Read the model definition and answer for the solid it produces. Units are mm, in the model's axes. A direction names the side the tool comes from. Round coordinates to 2 decimals unless told otherwise and drop trailing zeros. Order: outer loops, then holes, each group sorted by start corner. A loop starts at its lowest first (then second) coordinate and runs counter-clockwise, first axis right, second up.
from build123d import *

# Parameters (mm, degrees)
F0_W     = 18
F0_H     = 43.2
F1_DEPTH = 1.6
F3_DEPTH = 1
F2_W     = 10.35191
F2_H     = 3.05466
F4_DEPTH = 3


with BuildPart() as f1:
    # F0 (on Top) → F1 (new body)
    with BuildSketch(Plane.XY):
        with Locations((0, -1.040964)):
            Rectangle(F0_W, F0_H)
    extrude(amount=F1_DEPTH)

    # F2 (on face) → F3 (join)
    with BuildSketch(Plane.XY.offset(1.6)):
        Polygon((-3.383941, -9.864242), (0, -13.744771), (3.521491, -9.864242), (0, -5.74118), align=None)
    extrude(amount=F3_DEPTH)

    # F2 (on face) → F4 (join)
    with BuildSketch(Plane.XY.offset(1.6)):
        with Locations((0.296766, 17.023522)):
            Rectangle(F2_W, F2_H)
    extrude(amount=F4_DEPTH)


solid = f1.part
Q1. A cutting plane is placed at D-D, the plane x = 1.5. Give the vertices of the cut face in (y, z), plus the area to 3 significant figures.
Outcome:
outline: (-22.64, 0) - (20.56, 0) - (20.56, 1.6) - (18.55, 1.6) - (18.55, 4.6) - (15.5, 4.6) - (15.5, 1.6) - (-7.5, 1.6) - (-7.5, 2.6) - (-12.09, 2.6) - (-12.09, 1.6) - (-22.64, 1.6) - close
area: 82.9 mm2
Q2. A cutting plane is placed at A-A, the plane x = 4.75. Give the vertices of the cut face in (y, z), plus the area to 3 significant figures.
Outcome:
outline: (-22.64, 0) - (20.56, 0) - (20.56, 1.6) - (18.55, 1.6) - (18.55, 4.6) - (15.5, 4.6) - (15.5, 1.6) - (-22.64, 1.6) - close
area: 78.3 mm2
Q3. For faces 4 (the face through (0, 15.496, 3)), 5 (the face through (0, -10, 2.6)), 6 (the face through (5.473, 17, 3)), 7 (the face through (1.74, -11.83, 2.09)), 8 (the face through (1.785, -7.832, 2.093)), determine the directions among +Z, -Z, +X, -X, +Y, -Y from which every point of the face is accessible in a straight line to the end or side of a thin tool.
Outcome:
face 4: +Z, +X, -X
face 5: +Z, +X, -X, -Y
face 6: +Z, +X, +Y, -Y
face 7: +Z, +X, -Y
face 8: +Z, +X
Q4. For a pull along Y with two mould halves and no side action, classify faces 1 (the face through (0, -1, 1.6)), 2 (the face through (-4.879, 17, 3)), 3 (the face through (0, 18.551, 3)) as released by +Y, released by -Y, zero draft, split by the parting line, or undercut.
Outcome:
face 1: undercut
face 2: zero draft
face 3: released by +Y
Q5. A cutting plane is placed at C-C, the plane z = 3.25. Give the vertices of the cut face in (x, y), plus the area to 3 significant figures.
Outcome:
outline: (-4.88, 15.5) - (5.47, 15.5) - (5.47, 18.55) - (-4.88, 18.55) - close
area: 31.6 mm2
Q6. A cutting plane is placed at B-B, the plane y = -9. Give the vertices of the cut face in (x, z).
Outcome:
outline: (-9, 0) - (9, 0) - (9, 1.6) - (2.78, 1.6) - (2.78, 2.6) - (-2.67, 2.6) - (-2.67, 1.6) - (-9, 1.6) - close
Q7. Straight lines are drawn through the part: probe 1 along Z at (x, y) = (-6.5, 8); probe 2 along Y at (x, z) = (4, 3.8); probe 3 along Y at (x, z) = (-1, 2.5). For each, find the intervals that lie inside material, in ascending order.
Outcome:
probe 1: z = 0 to 1.6
probe 2: y = 15.5 to 18.55
probe 3: y = -12.6 to -6.96, 15.5 to 18.55
Q8. Flat-ended cylindrical pins translate along their axes: pin 1 (2 mm diameter, centred on x = 5, y = -1, fed in from +Z); pin 2 (5 mm diameter, centred on x = 0.5, y = -15.5, fed in from +Z); pin 3 (1.5 mm diameter, centred on y = 17, z = 3, fed in from +X). Find the tip coordinate at first contact, or state that the pin passes through.
Outcome:
pin 1: stops at z = 1.6
pin 2: stops at z = 2.6
pin 3: stops at x = 5.47
